Design review of the part built by this model. Coordinates are the model's own, in mm. Face numbers are marked on the shaded views. A direction names the side the tool comes from. Coordinates: 2 decimals unless noted, no trailing zeros. Write each loop counter-clockwise with the first axis right and the second up, starting at its lowest first coordinate (ties: lowest second). Pieces come first, ordered by that corner, then holes.
Q1. Machinability: for the marked faces 1 and 2, which of the approach directions +Z, -Z, +X, -X, +Y, -Y give a long, thin tool a straight path to every point of the face, cutting with its end or side? Answer none if there is none.
Q2. To check wall thickness, follow probe 1 along Y at (x, z) = (-20, 17.5); probe 2 along X at (y, z) = (56.5, -64.5); probe 3 along X at (y, z) = (3, -33). State the ranges of each line that lie inside material, in increasing order.
Q3. Add section C-C, the plane y = 12. Give the boundary of the cut face in (x, z), plus the area to 3 significant figures.
Q4. Add section A-A, the plane z = 0. Give the boundary of the cut face in (x, y) (3 decimals), plus the area to 3 significant figures.
Q5. Add section B-B, the plane x = -9. Give the boundary of the cut face in (y, z).
Q6. Clearance check with flat-ended pins moving along their axes: pin 1 Ø1.5 at (y, z) = (71, 0.5) entering from -X; pin 2 Ø23.5 at (x, y) = (7, 7.5) entering from +Z; pin 3 Ø23.5 at (x, y) = (11.5, 6) entering from -Z. State where each tip first meets the part, or that it passes through.
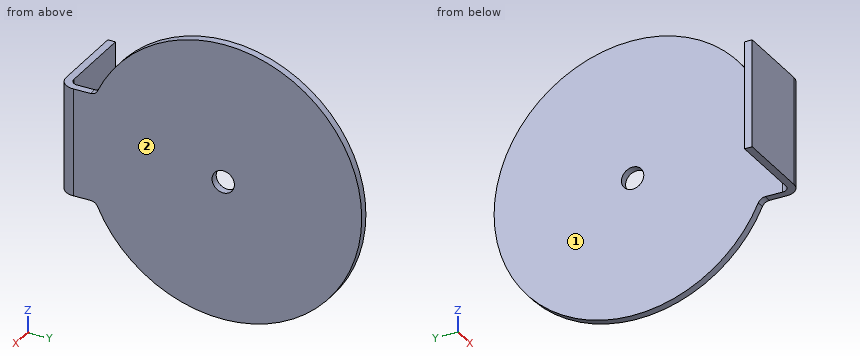
from build123d import *

# Parameters (mm, degrees)
ESBO_O1_W                      = 60
ESBO_O1_H                      = 70
FLANGE_BASE1_DEPTH             = 5
ARESTA_FLANGE1_STRIP_W         = 30
ARESTA_FLANGE1_STRIP_H         = 5
ARESTA_FLANGE1_STRIP_CUT_DEPTH = 70
ARESTA_FLANGE1_DEPTH           = 70
ESBO_O9_R                      = 90
ABA1_DEPTH                     = 5
FILETE5_R                      = 5
FILETE6_R                      = 5
ESBO_O10_R                     = 7.25
CORTE_EXTRUS_O1_DEPTH          = 5


# Sheet-metal steps are written as plain solids
with BuildPart() as part:
    # Esboço1 → Flange-base1 (new body)
    with BuildSketch(Plane(origin=(0, 0, 0), x_dir=(1, 0, 0), z_dir=(0, 1, 0))):
        Rectangle(ESBO_O1_W, ESBO_O1_H)
    extrude(amount=-FLANGE_BASE1_DEPTH)

    # Aresta-Flange1 strip (across the edge) → Aresta-Flange1 strip cut (cut)
    with BuildSketch(Plane(origin=(30, 0, 35), x_dir=(-1, 0, 0), z_dir=(0, 0, -1))):
        with Locations((-5, -2.5)):
            Rectangle(ARESTA_FLANGE1_STRIP_W, ARESTA_FLANGE1_STRIP_H)
    extrude(amount=ARESTA_FLANGE1_STRIP_CUT_DEPTH, mode=Mode.SUBTRACT)

    # Aresta-Flange1 section (across the edge) → Aresta-Flange1 (add)
    with BuildSketch(Plane(origin=(30, 0, 35), x_dir=(-1, 0, 0), z_dir=(0, 0, -1))):
        with BuildLine():
            Line((0, 5), (0, 86))
            Line((0, 86), (5, 86))
            Line((5, 86), (5, 5))
            ThreePointArc((5, 5), (6.464466094, 1.464466094), (10, 0))
            Line((10, 0), (10, -5))
            ThreePointArc((10, -5), (2.928932188, -2.071067812), (0, 5))
        make_face()
    extrude(amount=ARESTA_FLANGE1_DEPTH)

    # Esboço9 → Aba1 (add)
    with BuildSketch(Plane(origin=(30, 0, 0), x_dir=(0, 0, -1), z_dir=(1, 0, 0))):
        with Locations((0, 102.425)):
            Circle(ESBO_O9_R)
    extrude(amount=-ABA1_DEPTH)

    # Filete5
    filete5_edges = [part.edges().sort_by_distance(p)[0] for p in [
        (27.5, 19.509380241, -35),
    ]]
    fillet(filete5_edges, radius=FILETE5_R)

    # Filete6
    filete6_edges = [part.edges().sort_by_distance(p)[0] for p in [
        (27.5, 19.509380241, 35),
    ]]
    fillet(filete6_edges, radius=FILETE6_R)

    # Esboço10 → Corte-extrusão1 (cut)
    with BuildSketch(Plane(origin=(30, 0, 0), x_dir=(0, 0, -1), z_dir=(1, 0, 0))):
        with Locations(Location((0, 102.425, 0), (0, 0, 90))):
            Circle(ESBO_O10_R)
    extrude(amount=-CORTE_EXTRUS_O1_DEPTH, mode=Mode.SUBTRACT)


solid = part.part
Here are the results:
1. face 1: +Z, -Z, -X, +Y
1. face 2: +Z, -Z, +X, +Y, -Y
2. probe 1: y = -5 to 0
2. probe 2: x = 25 to 30
2. probe 3: x = 24.58 to 29.8
3. outline: (25, -35) - (30, -35) - (30, 35) - (25, 35) - close
3. area: 350 mm2
4. outline: (-30, -5) - (20, -5) arc R10 ccw to (30, 5) - (30, 95.175) - (25, 95.175) - (25, 5) arc R5 cw to (20, 0) - (-30, 0) - close; (25, 109.675) - (30, 109.675) - (30, 192.425) - (25, 192.425) - close
4. area: 1,170 mm2
5. outline: (-5, -35) - (0, -35) - (0, 35) - (-5, 35) - close
6. pin 1: stops at x = 25
6. pin 2: stops at z = 35
6. pin 3: stops at z = -35
